Part model, mm, in its own coordinate system. A direction names the side the tool comes from. Round coordinates to 2 decimals unless told otherwise and drop trailing zeros. Order: outer loops, then holes, each group sorted by start corner. A loop starts at its lowest first (then second) coordinate and runs counter-clockwise, first axis right, second up. Notation, with made-up numbers: M 20.25,-3 L 26.25,-3 A5 cw 26.25,3 Z; hole C 10.25,45 d2. An arc over 180 degrees is marked long. One line per question, with ' | ' between items.
from build123d import *

# Parameters (mm, degrees)
F0_W      = 6
F0_H      = 5
F0_W_2    = 1.2
F1_DEPTH  = 1.2
F2_DEPTH  = 5
F3_DEPTH  = 10
F5_DEPTH  = 65
F6_DEPTH  = 10
F1_FACE_W = 78.9
F1_FACE_H = 1.2
F7_DEPTH  = 16.3
F8_DEPTH  = 16.4


with BuildPart() as f1:
    # F0 (on Top) → F1 (new body)
    with BuildSketch(Plane.XY):
        with Locations((14.2, -2.5)):
            Rectangle(F0_W, F0_H)
        with Locations((10.6, -2.5)):
            Rectangle(F0_W_2, F0_H)
        Polygon((10, 0), (0, 0), (0, -76.2), (78.9, -76.2), (78.9, 0), (68.9, 0), (68.9, -5), (67.7, -5), (61.7, -5), (61.7, 0), (17.2, 0), (17.2, -5), (11.2, -5), (10, -5), align=None)
        Polygon((10, -60), (11.2, -60), (17.2, -60), (17.2, -65), (17.2, -66.2), (10, -66.2), align=None, mode=Mode.SUBTRACT)
        Polygon((61.7, -65), (61.7, -60), (67.7, -60), (68.9, -60), (68.9, -66.2), (61.7, -66.2), align=None, mode=Mode.SUBTRACT)
        with Locations((64.7, -2.5)):
            Rectangle(F0_W, F0_H)
        with Locations((68.3, -2.5)):
            Rectangle(F0_W_2, F0_H)
        with Locations((64.7, -62.5)):
            Rectangle(F0_W, F0_H)
        Polygon((68.9, -60), (67.7, -60), (67.7, -65), (61.7, -65), (61.7, -66.2), (68.9, -66.2), align=None)
        with Locations((14.2, -62.5)):
            Rectangle(F0_W, F0_H)
        Polygon((11.2, -65), (11.2, -60), (10, -60), (10, -66.2), (17.2, -66.2), (17.2, -65), align=None)
    extrude(amount=-F1_DEPTH)

    # F0 (on Top) → F2 (join)
    with BuildSketch(Plane.XY):
        with Locations((14.2, -2.5)):
            Rectangle(F0_W, F0_H)
        with Locations((14.2, -62.5)):
            Rectangle(F0_W, F0_H)
        with Locations((64.7, -2.5)):
            Rectangle(F0_W, F0_H)
        with Locations((64.7, -62.5)):
            Rectangle(F0_W, F0_H)
    extrude(amount=F2_DEPTH)

    # F0 (on Top) → F3 (join)
    with BuildSketch(Plane.XY):
        Polygon((11.2, -65), (11.2, -60), (10, -60), (10, -66.2), (17.2, -66.2), (17.2, -65), align=None)
        Polygon((68.9, -60), (67.7, -60), (67.7, -65), (61.7, -65), (61.7, -66.2), (68.9, -66.2), align=None)
        with Locations((68.3, -2.5)):
            Rectangle(F0_W_2, F0_H)
        with Locations((10.6, -2.5)):
            Rectangle(F0_W_2, F0_H)
    extrude(amount=F3_DEPTH)

    # F4 (on face) → F5 (join, through all)
    with BuildSketch(Plane(origin=(0, 0, 0), x_dir=(-1, 0, 0), z_dir=(0, 1, 0))):
        Polygon((-11.2, 6), (-11.2, 10), (-12.7, 8.5), (-12.7, 7.5), align=None)
        Polygon((-66.2, 7.5), (-66.2, 8.5), (-67.7, 10), (-67.7, 6), align=None)
    extrude(amount=-F5_DEPTH)

    # F0 (on Top) → F6 (cut, through all)
    with BuildSketch(Plane.XY):
        Polygon((10, 0), (0, 0), (0, -76.2), (78.9, -76.2), (78.9, 0), (68.9, 0), (68.9, -5), (67.7, -5), (61.7, -5), (61.7, 0), (17.2, 0), (17.2, -5), (11.2, -5), (10, -5), align=None)
        Polygon((10, -60), (11.2, -60), (17.2, -60), (17.2, -65), (17.2, -66.2), (10, -66.2), align=None, mode=Mode.SUBTRACT)
        Polygon((61.7, -65), (61.7, -60), (67.7, -60), (68.9, -60), (68.9, -66.2), (61.7, -66.2), align=None, mode=Mode.SUBTRACT)
    extrude(amount=F6_DEPTH, mode=Mode.SUBTRACT)

    # F1_face (on face) → F7 (join)
    with BuildSketch(Plane(origin=(39.45, -76.2, -0.6), x_dir=(1, 0, 0), z_dir=(0, -1, 0))):
        Rectangle(F1_FACE_W, F1_FACE_H)
    extrude(amount=F7_DEPTH)

    # F5_face (on face) → F8 (join)
    with BuildSketch(Plane(origin=(39.45, 0, 1.467354), x_dir=(-1, 0, 0), z_dir=(0, 1, 0))):
        Polygon((-39.45, -2.667354), (39.45, -2.667354), (39.45, -1.467354), (29.45, -1.467354), (29.45, 8.532646), (28.25, 8.532646), (26.75, 7.032646), (26.75, 6.032646), (28.25, 4.532646), (28.25, 3.532646), (22.25, 3.532646), (22.25, -1.467354), (-22.25, -1.467354), (-22.25, 3.532646), (-28.25, 3.532646), (-28.25, 4.532646), (-26.75, 6.032646), (-26.75, 7.032646), (-28.25, 8.532646), (-29.45, 8.532646), (-29.45, -1.467354), (-39.45, -1.467354), align=None)
    extrude(amount=F8_DEPTH)


solid = f1.part
1) Which spindle directions (+Z, -Z, +X, -X, +Y, -Y) get a long thin tool onto all of the face, cutting with end or side? Do faces 1 (the face through (10, 6, 5)), 2 (the face through (61.7, 6, 2)), 3 (the face through (65, 6, 5)), 4 (the face through (66, -5, 4)), 5 (the face through (14, -66.2, 5)). Say none if no direction does.
The answers:
face 1: +Z, -X, +Y, -Y | face 2: +Z, +Y, -Y | face 3: +Y | face 4: +Z, +X, -X | face 5: +Z, +X, -X, -Y
2) Saw through at B-B (y = -62). List the corners of the cut face in (x, z), plus the area to 3 significant figures.
The answers:
outline: M 0,-1.2 L 78.9,-1.2 L 78.9,0 L 68.9,0 L 68.9,10 L 67.7,10 L 66.2,8.5 L 66.2,7.5 L 67.7,6 L 67.7,5 L 61.7,5 L 61.7,0 L 17.2,0 L 17.2,5 L 11.2,5 L 11.2,6 L 12.7,7.5 L 12.7,8.5 L 11.2,10 L 10,10 L 10,0 L 0,0 Z | area: 186 mm²
3) Saw through at A-A (z = 2.25). List the corners of the cut face in (x, y).
The answers:
outline: M 10,-66.2 L 17.2,-66.2 L 17.2,-60 L 10,-60 Z; M 10,-5 L 17.2,-5 L 17.2,16.4 L 10,16.4 Z; M 61.7,-66.2 L 68.9,-66.2 L 68.9,-60 L 61.7,-60 Z; M 61.7,-5 L 68.9,-5 L 68.9,16.4 L 61.7,16.4 Z
4) Probe line 1 (X direction, y = 6, z = 3); line 2 (X direction, y = -1.5, z = 7.5); line 3 (Z direction, x = 29.5, y = -81). List the from-to ranges inside material, lowest first. Write a range as [from, to].
The answers:
line 1: x = [10, 17.2], [61.7, 68.9] | line 2: x = [10, 12.7], [66.2, 68.9] | line 3: z = [-1.2, 0]
5) Saw through at D-D (y = -10). List the corners of the cut face in (x, z).
The answers:
outline: M 0,-1.2 L 78.9,-1.2 L 78.9,0 L 0,0 Z
6) Two-plate mould, pull along Z, no slides. Class faces 6 (the face through (40, -39, -1.2)), 7 (the face through (65, -66.2, 5)), 8 (the face through (14, -62, 5)): released by +Z, released by -Z, zero draft, split by the parting line, or undercut.
The answers:
face 6: released by -Z | face 7: zero draft | face 8: undercut
7) Saw through at C-C (x = 43). List the corners of the cut face in (y, z).
The answers:
outline: M -92.5,-1.2 L 16.4,-1.2 L 16.4,0 L -92.5,0 Z
8) Drop flat-ended pins along their axis: pin 1 (4 mm diameter, centred on y = 1.5, z = 4, fed in from +X); pin 2 (3.5 mm diameter, centred on x = 66.5, z = 4, fed in from -Y); pin 3 (1.5 mm diameter, centred on x = 61, y = -46.5, fed in from +Z). Give the stop position or say it passes through.
The answers:
pin 1: stops at x = 68.9 | pin 2: stops at y = -66.2 | pin 3: stops at z = 0
